Geometry: final body of the model. Coordinates: model frame, mm. A direction names the side the tool comes from. Give positions to 0.01 mm unless a question says otherwise; leave off trailing zeros. Write each loop counter-clockwise with the first axis right and the second up, starting at its lowest first coordinate (ties: lowest second). Pieces come first, ordered by that corner, then holes. Notation, with made-up numbers: (3.25, 58.5) -> (62.25, 58.5) arc R36 cw to (62.25, 93.5) -> close; hole circle Ø4 at (10.25, 52.25). An arc over 180 degrees is marked (long way). Answer in a Markdown table with one row per item. Add a question column.
Item 1: Draft query along X for faces 5 (the cylindrical face through (-20.974, 0.481, 0.056)), 6 (the flat face through (4.317, 7.854, 0.063)), 7 (the flat face through (20, 7, 4.5)), 8 (the flat face through (-37.5, -4, 0)). Return one class per face: +X half, -X half, draft (parallel to the pull), parting line (faces both ways), or undercut.
Item 2: Material intervals for probe 1 along Z at (x, y) = (-37, -16.5); probe 2 along Z at (x, y) = (-45.5, -8.5); probe 3 along Y at (x, z) = (-44.5, 15.6), sorted ascending. Write a range as from..to.
Item 3: First-contact query: P1, Ø0.8, axis at x = -4, z = -4.5, coming from the -Y side; P2, Ø1.5, axis at x = -30.5, z = -1.5, coming from the -Y side; P3, Ø4, axis at y = -2, z = -12.5, coming from the +X side. Flat tips, straight axial feed; report the tip coordinate or a pass-through.
Item 4: Section query B-B on x = -44.5. Output: boundary loops of the cut face in (y, z), plus the area to 3 significant figures.
Item 5: Access query for faces 1 (the flat face through (0, -6, 0)), 2 (the flat face through (8.7, -5.7, 5)), 3 (the flat face through (-19.245, 7.854, 0.063)), 4 (the flat face through (-9, 7, -4.5)). Directions: +Z, -Z, +X, -X, +Y, -Y. A direction counts if a zero-diameter tool reaches every point of the face in a straight line with its end or side. Return the directions, or none.
Item 6: Section query A-A on y = -10.5. Output: boundary loops of the cut face in (x, z).
Item 7: Section query C-C on y = -16. Output: boundary loops of the cut face in (x, z), plus the area to 3 significant figures.
Item 8: Section query D-D on z = 15.5. Output: boundary loops of the cut face in (x, y), plus the area to 3 significant figures.
```python
from build123d import *

# Parameters (mm, degrees)
MAIN_EXTRUSION_DEPTH          = 5
TOOTH_DEPTH                   = 4.5
TOOTH_FILLET_R                = 0.57
TOOTHREPEAT_COUNT             = 9
TOOTHREPEAT_PITCH             = 4.71238898
TOOTH_FILLET_OF_TOOTHREPEAT_R = 0.57
FIXINGSUPPORT_DEPTH           = 28
ESQUISSE11_R                  = 2.6
FIXINGHOLES_DEPTH             = 64.832671885
ESQUISSE12_W                  = 15
ESQUISSE12_H                  = 12
RACKHOLE_DEPTH                = 67.767057746
FILLET_2_DEPTH                = 16
ESQUISSE15_W                  = 50
ESQUISSE15_H                  = 10.2
REINFORCEMENT_DEPTH           = 1
ESQUISSE16_R                  = 1.6
ENL_V_MAT_EXTRU_2_DEPTH       = 58.798702408


with BuildPart() as part:
    # Esquisse1 → Main Extrusion (new, symmetric)
    with BuildSketch(Plane.XY):
        with BuildLine():
            Line((-22.5, 6), (-27.5, 7))
            Line((-27.5, 7), (-32.5, 7))
            Line((-32.5, 7), (-32.5, -7))
            Line((-32.5, -7), (-27.5, -7))
            Line((-27.5, -7), (-22.5, -6))
            Line((-22.5, -6), (22.5, -6))
            ThreePointArc((22.5, -6), (28.5, 0), (22.5, 6))
            Line((22.5, 6), (-22.5, 6))
        make_face()
    extrude(amount=MAIN_EXTRUSION_DEPTH, both=True)

    # Esquisse5 → Tooth (add, symmetric)
    with BuildSketch(Plane.XY):
        Polygon((17.778917131, 6), (19.007316672, 9.375), (20.271600459, 9.375), (21.5, 6), align=None)
    tooth = extrude(amount=TOOTH_DEPTH, both=True)

    # Tooth Fillet
    tooth_fillet_edges = [part.edges().sort_by_distance(p)[0] for p in [
        (17.778917131, 6, 0),
        (21.5, 6, 0),
    ]]
    fillet(tooth_fillet_edges, radius=TOOTH_FILLET_R)

    # ToothRepeat: Tooth ×9
    with Locations(*[(-i * TOOTHREPEAT_PITCH, 0, 0) for i in range(1, TOOTHREPEAT_COUNT)]):
        add(tooth)

    # Tooth Fillet of ToothRepeat
    tooth_fillet_of_toothrepeat_edges = [part.edges().sort_by_distance(p)[0] for p in [
        (13.066528151, 6, 0),
        (16.78761102, 6, 0),
        (8.354139171, 6, 0),
        (12.07522204, 6, 0),
        (3.641750191, 6, 0),
        (7.36283306, 6, 0),
        (-1.070638789, 6, 0),
        (2.65044408, 6, 0),
        (-5.783027769, 6, 0),
        (-2.0619449, 6, 0),
        (-10.495416749, 6, 0),
        (-6.77433388, 6, 0),
        (-15.207805729, 6, 0),
        (-11.48672286, 6, 0),
        (-19.920194709, 6, 0),
        (-16.19911184, 6, 0),
    ]]
    fillet(tooth_fillet_of_toothrepeat_edges, radius=TOOTH_FILLET_OF_TOOTHREPEAT_R)



with BuildPart() as body_2:
    # Esquisse10 → FixingSupport (new body)
    with BuildSketch(Plane(origin=(0, 7, 0), x_dir=(1, 0, 0), z_dir=(0, 1, 0))):
        Polygon((-32.5, -17.2), (-49.5, -17.2), (-49.5, -12.2), (-37.5, -12.2), (-37.5, 12.2), (-49.5, 12.2), (-49.5, 17.2), (-32.5, 17.2), align=None)
    extrude(amount=-FIXINGSUPPORT_DEPTH)

    # Esquisse11 → FixingHoles (cut, through all)
    with BuildSketch(Plane.XY.offset(17.2)):
        with Locations((-44.5, -16)):
            Circle(ESQUISSE11_R)
    extrude(amount=-FIXINGHOLES_DEPTH, mode=Mode.SUBTRACT)

    # Esquisse12 → RackHole (cut, through all)
    with BuildSketch(Plane(origin=(-32.5, 0, 0), x_dir=(0, 0, -1), z_dir=(1, 0, 0))):
        with Locations((0, -15)):
            Rectangle(ESQUISSE12_W, ESQUISSE12_H)
    extrude(amount=-RACKHOLE_DEPTH, mode=Mode.SUBTRACT)


with BuildPart() as part_1:
    add(part.part)

    add(body_2.part)  # Fillet 2 merges body 2
    # Esquisse14 → Fillet 2 (add)
    with BuildSketch(Plane(origin=(0, 7, 0), x_dir=(1, 0, 0), z_dir=(0, 1, 0))):
        with BuildLine():
            Line((-32.5, -5), (-32.5, -10))
            ThreePointArc((-32.5, -10), (-31.035533906, -6.464466094), (-27.5, -5))
            Line((-27.5, -5), (-32.5, -5))
        make_face()
    fillet_2 = extrude(amount=-FILLET_2_DEPTH)

    # FilletSymetry: Fillet 2 across plane
    add(fillet_2.mirror(Plane.XY))

    # Esquisse15 → Reinforcement (cut)
    with BuildSketch(Plane.XY.offset(5)):
        with Locations((-2.5, 0)):
            Rectangle(ESQUISSE15_W, ESQUISSE15_H)
    reinforcement = extrude(amount=-REINFORCEMENT_DEPTH, mode=Mode.SUBTRACT)

    # Symétrie1: Reinforcement across plane
    add(reinforcement.mirror(Plane.XY), mode=Mode.SUBTRACT)

    # Esquisse16 → Enlèv. mat.-Extru.2 (cut, through all)
    with BuildSketch(Plane.XY.offset(4)):
        with Locations((17.5, 0)):
            Circle(ESQUISSE16_R)
        with Locations((7.5, 0)):
            Circle(ESQUISSE16_R)
        with Locations((-2.5, 0)):
            Circle(ESQUISSE16_R)
        with Locations((-12.5, 0)):
            Circle(ESQUISSE16_R)
        with Locations((-22.5, 0)):
            Circle(ESQUISSE16_R)
    extrude(amount=-ENL_V_MAT_EXTRU_2_DEPTH, mode=Mode.SUBTRACT)


solid = part_1.part
```
Findings below:
| question | item | result |
|---|---|---|
| 1 | face 5 | undercut |
| 1 | face 6 | undercut |
| 1 | face 7 | draft |
| 1 | face 8 | -X half |
| 2 | probe 1 | z = -17.2..-7.5, 7.5..17.2 |
| 2 | probe 2 | z = -17.2..-12.2, 12.2..17.2 |
| 2 | probe 3 | y = -21..-18.6, -13.4..7 |
| 3 | P1 | stops at y = -6 |
| 3 | P2 | stops at y = -7 |
| 3 | P3 | stops at x = -32.5 |
| 4 | outline | (-21, -17.2) -> (-18.6, -17.2) -> (-18.6, -12.2) -> (-21, -12.2) -> close; (-21, 12.2) -> (-18.6, 12.2) -> (-18.6, 17.2) -> (-21, 17.2) -> close; (-13.4, -17.2) -> (7, -17.2) -> (7, -12.2) -> (-13.4, -12.2) -> close; (-13.4, 12.2) -> (7, 12.2) -> (7, 17.2) -> (-13.4, 17.2) -> close |
| 4 | area | 228 mm^2 |
| 5 | face 1 | +Z, -Z, +X, -Y |
| 5 | face 2 | +Z, +X, +Y, -Y |
| 5 | face 3 | +Z, -Z, +Y |
| 5 | face 4 | -Z, +X, +Y |
| 6 | outline | (-49.5, -17.2) -> (-32.5, -17.2) -> (-32.5, -7.5) -> (-37.5, -7.5) -> (-37.5, -12.2) -> (-49.5, -12.2) -> close; (-49.5, 12.2) -> (-37.5, 12.2) -> (-37.5, 7.5) -> (-32.5, 7.5) -> (-32.5, 17.2) -> (-49.5, 17.2) -> close |
| 7 | outline | (-49.5, -17.2) -> (-47.1, -17.2) -> (-47.1, -12.2) -> (-49.5, -12.2) -> close; (-49.5, 12.2) -> (-47.1, 12.2) -> (-47.1, 17.2) -> (-49.5, 17.2) -> close; (-41.9, -17.2) -> (-32.5, -17.2) -> (-32.5, -7.5) -> (-37.5, -7.5) -> (-37.5, -12.2) -> (-41.9, -12.2) -> close; (-41.9, 12.2) -> (-37.5, 12.2) -> (-37.5, 7.5) -> (-32.5, 7.5) -> (-32.5, 17.2) -> (-41.9, 17.2) -> close |
| 7 | area | 165 mm^2 |
| 8 | outline | (-49.5, -21) -> (-32.5, -21) -> (-32.5, 7) -> (-49.5, 7) -> close; hole circle Ø5.2 at (-44.5, -16) |
| 8 | area | 455 mm^2 |
